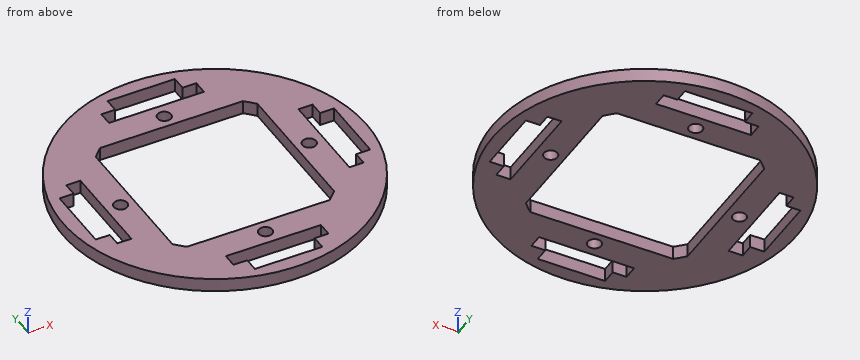
from build123d import *

# Parameters (mm, degrees)
SKETCH_1_R      = 22.5
EXTRUDE_1_DEPTH = 2
MM_1_D          = 2
MM_1_DEPTH      = 5.2
MM_1_TIP        = 0.600860619


with BuildPart() as part:
    # 草图1 → 凸台-拉伸1 (new body)
    with BuildSketch(Plane.XY):
        Circle(SKETCH_1_R)
        with BuildLine():
            Line((10.583005244, -12), (-10.583005244, -12))
            ThreePointArc((-10.583005244, -12), (-11.313708499, -11.313708499), (-12, -10.583005244))
            Line((-12, -10.583005244), (-12, 10.583005244))
            ThreePointArc((-12, 10.583005244), (-11.313708499, 11.313708499), (-10.583005244, 12))
            Line((-10.583005244, 12), (10.583005244, 12))
            ThreePointArc((10.583005244, 12), (11.313708499, 11.313708499), (12, 10.583005244))
            Line((12, 10.583005244), (12, -10.583005244))
            ThreePointArc((12, -10.583005244), (11.313708499, -11.313708499), (10.583005244, -12))
        make_face(mode=Mode.SUBTRACT)
        Polygon((-5, 18.275), (-5, 20.375), (5, 20.375), (5, 18.275), (7.05, 18.275), (7.05, 16.175), (-7.05, 16.175), (-7.05, 18.275), align=None, mode=Mode.SUBTRACT)
        Polygon((-18.275, 7.05), (-16.175, 7.05), (-16.175, -7.05), (-18.275, -7.05), (-18.275, -5), (-20.375, -5), (-20.375, 5), (-18.275, 5), align=None, mode=Mode.SUBTRACT)
        Polygon((-7.05, -18.275), (-7.05, -16.175), (7.05, -16.175), (7.05, -18.275), (5, -18.275), (5, -20.375), (-5, -20.375), (-5, -18.275), align=None, mode=Mode.SUBTRACT)
        Polygon((18.275, -7.05), (16.175, -7.05), (16.175, 7.05), (18.275, 7.05), (18.275, 5), (20.375, 5), (20.375, -5), (18.275, -5), align=None, mode=Mode.SUBTRACT)
    extrude(amount=EXTRUDE_1_DEPTH)

    # 大小mm 暗销孔1
    with Locations(Plane.XY.offset(2)):
        with Locations((0, 14), (-14, 0), (0, -14), (14, 0)):
            Hole(MM_1_D / 2, depth=MM_1_DEPTH)
            with Locations((0, 0, -(MM_1_DEPTH + MM_1_TIP / 2))):  # 118° drill point
                Cone(0, MM_1_D / 2, MM_1_TIP, mode=Mode.SUBTRACT)


solid = part.part
CAD build for the part. Positions are in the model's coordinates, mm. Coordinates: 2 decimals unless noted, no trailing zeros. Order: outer loops, then holes, each group sorted by start corner. A loop starts at its lowest first (then second) coordinate and runs counter-clockwise, first axis right, second up. Notation, with made-up numbers: (-20.75, -24.75) -> (36.25, -24.75) arc R16 ccw to (36.25, 6.25) -> close; hole circle Ø10 at (16, 32.25). An arc over 180 degrees is marked (long way). Answer in a Markdown table with one row per item.
1) Band-saw the part on A-A (y = 0). List the corners of the cut face in (x, z) (3 decimals), and give its area (3 significant figures).
Check values:
| item | result |
|---|---|
| outline | (-22.5, 0) -> (-20.375, 0) -> (-20.375, 2) -> (-22.5, 2) -> close; (-16.175, 0) -> (-15, 0) -> (-15, 2) -> (-16.175, 2) -> close; (-13, 0) -> (-12, 0) -> (-12, 2) -> (-13, 2) -> close; (12, 0) -> (13, 0) -> (13, 2) -> (12, 2) -> close; (15, 0) -> (16.175, 0) -> (16.175, 2) -> (15, 2) -> close; (20.375, 0) -> (22.5, 0) -> (22.5, 2) -> (20.375, 2) -> close |
| area | 17.2 mm2 |
2) Flat gauge pins, fed straight in: P1, Ø0.6, axis at x = 17.5, z = 1, coming from the -Y side; P2, Ø1, axis at x = 15.5, z = 1, coming from the +Y side; P3, Ø0.6, axis at x = 16.5, z = 1, coming from the +Y side; P4, Ø1.6, axis at x = -14, y = 0, coming from the -Z side. Where does each tip first touch, or does it go through?
Check values:
| item | result |
|---|---|
| P1 | y = -14.51 |
| P2 | y = 16.77 |
| P3 | y = 15.61 |
| P4 | through |
3) Drill centre lines: line 1 (Y direction, x = 0, z = 1.45) (3 decimals); line 2 (Y direction, x = 3, z = 0.85) (3 decimals); line 3 (Y direction, x = 19.5, z = 1.5). Where is each one in solid material? Low to high.
Check values:
| item | result |
|---|---|
| line 1 | -22.5 to -20.375, -16.175 to -15, -13 to -12, 12 to 13, 15 to 16.175, 20.375 to 22.5 |
| line 2 | -22.299 to -20.375, -16.175 to -12, 12 to 16.175, 20.375 to 22.299 |
| line 3 | -11.22 to -5, 5 to 11.22 |
4) Band-saw the part on C-C (y = -14). List the corners of the cut face in (x, z), and give its area (3 significant figures).
Check values:
| item | result |
|---|---|
| outline | (-17.61, 0) -> (-1, 0) -> (-1, 2) -> (-17.61, 2) -> close; (1, 0) -> (17.61, 0) -> (17.61, 2) -> (1, 2) -> close |
| area | 66.5 mm2 |
